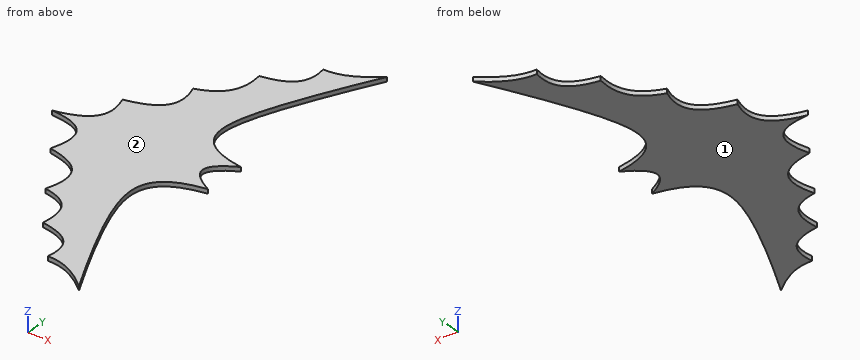
Autodesk Fusion 360 part; units mm, degrees
sketch "Sketch1" plane through (0, 0, 0) normal (0, 0, 1) x (1, 0, 0)
  spline S0 degree 5 poles (20, 5) (19.6208, 4.8) (18.8954, 4.4) (17.9067, 3.8) (16.7905, 3) (15.7547, 2) (15.1106, 1) (14.89, 0) (15.1106, -1) (15.7547, -2) (16.7905, -3) (17.9067, -3.8) (18.8954, -4.4) (19.6208, -4.8) (20, -5) knots 0 0 0 0 0 0 0.1 0.2 0.3 0.4 0.5 0.6 0.7 0.8 0.9 1 1 1 1 1 1
  spline S1 degree 5 poles (20, 5) (19.2712, 5.1081) (17.8733, 5.3538) (15.9554, 5.8111) (13.759, 6.5997) (11.6261, 7.8912) (10.1129, 9.4979) (9.2114, 11.428) (8.8832, 13.6833) (9.0671, 16.2602) (9.6928, 19.1509) (10.6903, 22.3442) (11.9999, 25.8244) (13.5744, 29.5733) (15.3779, 33.5733) (17.3852, 37.8091) (19.1413, 41.3771) (20.5394, 44.1509) (21.5072, 46.0431) (22, 47) knots 0 0 0 0 0 0 0.066667 0.133333 0.2 0.266667 0.333333 0.4 0.466667 0.533333 0.6 0.666667 0.733333 0.8 0.866667 0.933333 1 1 1 1 1 1
  spline S2 degree 5 poles (20, -5) (19.2712, -5.1081) (17.8733, -5.3538) (15.9554, -5.8111) (13.759, -6.5997) (11.6261, -7.8912) (10.1129, -9.4979) (9.2114, -11.428) (8.8832, -13.6833) (9.0671, -16.2602) (9.6928, -19.1509) (10.6903, -22.3442) (11.9999, -25.8244) (13.5744, -29.5733) (15.3779, -33.5733) (17.3852, -37.8091) (19.1413, -41.3771) (20.5394, -44.1509) (21.5072, -46.0431) (22, -47) knots 0 0 0 0 0 0 0.066667 0.133333 0.2 0.266667 0.333333 0.4 0.466667 0.533333 0.6 0.666667 0.733333 0.8 0.866667 0.933333 1 1 1 1 1 1
  spline S3 degree 5 poles (22, 47) (21.7727, 46.8021) (21.3189, 46.4146) (20.6399, 45.8581) (19.7383, 45.1666) (18.6179, 44.3921) (17.5049, 43.7166) (16.4, 43.1495) (15.3036, 42.6985) (14.2158, 42.3629) (13.136, 42.1358) (12.2781, 42.0345) (11.6378, 42.001) (11.2124, 41.9972) (11, 42) knots 0 0 0 0 0 0 0.1 0.2 0.3 0.4 0.5 0.6 0.7 0.8 0.9 1 1 1 1 1 1
  spline S4 degree 5 poles (22, -47) (21.7727, -46.8021) (21.3189, -46.4146) (20.6399, -45.8581) (19.7383, -45.1666) (18.6179, -44.3921) (17.5049, -43.7166) (16.4, -43.1495) (15.3036, -42.6985) (14.2158, -42.3629) (13.136, -42.1358) (12.2781, -42.0345) (11.6378, -42.001) (11.2124, -41.9972) (11, -42) knots 0 0 0 0 0 0 0.1 0.2 0.3 0.4 0.5 0.6 0.7 0.8 0.9 1 1 1 1 1 1
  spline S5 degree 5 poles (11, 42) (11.0567, 41.6874) (11.1508, 41.074) (11.2338, 40.1895) (11.2264, 39.0824) (11.0075, 37.8268) (10.5616, 36.7102) (9.8726, 35.7422) (8.9361, 34.9257) (7.7664, 34.252) (6.3831, 33.7089) (5.1205, 33.3698) (4.0916, 33.1657) (3.3698, 33.0516) (3, 33) knots 0 0 0 0 0 0 0.1 0.2 0.3 0.4 0.5 0.6 0.7 0.8 0.9 1 1 1 1 1 1
  spline S6 degree 5 poles (11, -42) (11.0567, -41.6874) (11.1508, -41.074) (11.2338, -40.1895) (11.2264, -39.0824) (11.0075, -37.8268) (10.5616, -36.7102) (9.8726, -35.7422) (8.9361, -34.9257) (7.7664, -34.252) (6.3831, -33.7089) (5.1205, -33.3698) (4.0916, -33.1657) (3.3698, -33.0516) (3, -33) knots 0 0 0 0 0 0 0.1 0.2 0.3 0.4 0.5 0.6 0.7 0.8 0.9 1 1 1 1 1 1
  spline S7 degree 5 poles (3, 33) (3.0488, 32.6643) (3.1298, 32.003) (3.2017, 31.0414) (3.1969, 29.8211) (3.0117, 28.4056) (2.6312, 27.1097) (2.0398, 25.9431) (1.2292, 24.9109) (0.2085, 24.0075) (-1.0064, 23.2232) (-2.1209, 22.683) (-3.0317, 22.3239) (-3.6718, 22.1046) (-4, 22) knots 0 0 0 0 0 0 0.1 0.2 0.3 0.4 0.5 0.6 0.7 0.8 0.9 1 1 1 1 1 1
  spline S8 degree 5 poles (3, -33) (3.0519, -32.6532) (3.1391, -31.9722) (3.2199, -30.9891) (3.2258, -29.756) (3.0522, -28.3533) (2.6811, -27.1017) (2.0958, -26.0139) (1.2865, -25.0975) (0.261, -24.3466) (-0.965, -23.749) (-2.0931, -23.3837) (-3.0168, -23.1691) (-3.6666, -23.052) (-4, -23) knots 0 0 0 0 0 0 0.1 0.2 0.3 0.4 0.5 0.6 0.7 0.8 0.9 1 1 1 1 1 1
  spline S9 degree 5 poles (-4, 22) (-3.8671, 21.6411) (-3.6275, 20.9356) (-3.3469, 19.9148) (-3.1327, 18.6296) (-3.149, 17.1578) (-3.4725, 15.8318) (-4.1248, 14.6617) (-5.1107, 13.6499) (-6.4105, 12.787) (-7.9976, 12.0604) (-9.4768, 11.5784) (-10.6963, 11.2692) (-11.5574, 11.0859) (-12, 11) knots 0 0 0 0 0 0 0.1 0.2 0.3 0.4 0.5 0.6 0.7 0.8 0.9 1 1 1 1 1 1
  spline S10 degree 5 poles (-4, -23) (-3.8615, -22.5957) (-3.6109, -21.8015) (-3.3142, -20.6538) (-3.0793, -19.2121) (-3.0716, -17.5674) (-3.3744, -16.0936) (-4.0114, -14.8039) (-4.9925, -13.7036) (-6.3007, -12.7834) (-7.91, -12.029) (-9.4177, -11.5468) (-10.6645, -11.249) (-11.5464, -11.0783) (-12, -11) knots 0 0 0 0 0 0 0.1 0.2 0.3 0.4 0.5 0.6 0.7 0.8 0.9 1 1 1 1 1 1
  spline S11 degree 5 poles (-12, 11) (-11.8671, 10.6411) (-11.6275, 9.9356) (-11.3469, 8.9148) (-11.1327, 7.6296) (-11.149, 6.1578) (-11.4725, 4.8318) (-12.1248, 3.6617) (-13.1107, 2.6499) (-14.4105, 1.787) (-15.9976, 1.0604) (-17.4768, 0.5784) (-18.6963, 0.2692) (-19.5574, 0.0859) (-20, 0) knots 0 0 0 0 0 0 0.1 0.2 0.3 0.4 0.5 0.6 0.7 0.8 0.9 1 1 1 1 1 1
  spline S12 degree 5 poles (-12, -11) (-11.8595, -10.5833) (-11.605, -9.7673) (-11.3024, -8.5952) (-11.0601, -7.1378) (-11.0439, -5.5036) (-11.3393, -4.0734) (-11.9708, -2.8631) (-12.9501, -1.8804) (-14.2612, -1.1149) (-15.8784, -0.5497) (-17.3964, -0.2443) (-18.653, -0.0926) (-19.5424, -0.0252) (-20, 0) knots 0 0 0 0 0 0 0.1 0.2 0.3 0.4 0.5 0.6 0.7 0.8 0.9 1 1 1 1 1 1
  point P0 (15, 0)
  point P1 (10, 10)
  point P2 (10, 20)
  point P3 (10, -10)
  point P4 (10, -20)
  point P5 (16, 43)
  point P6 (16, -43)
  point P7 (10, 36)
  point P8 (10, -36)
  point P9 (2, 26)
  point P10 (2, -26)
  point P11 (-4, 15)
  point P12 (-4, -15)
  point P13 (-12, 4)
  point P14 (-12, -3)
extrude "Extrude1" add sketch "Sketch1" along normal blind 1
CAD build for the part. Positions are in the model's coordinates, mm. Face numbers are marked on the shaded views. Give positions to 0.01 mm unless a question says otherwise; leave off trailing zeros.
(1) Saw through at A-A, the plane x = 17.5. State how many separate pieces and enclosed holes the cut face has, then the cut area to 3 significant figures.
(2) Drill centre lines: L1, parallel to X at y = 31, z = 0.6; L2, parallel to Y at x = -13, z = 0.4; L3, parallel to X at y = 28, z = 0.4. Where is each one in solid material? Low to high.
(3) Mould opens along Z. For the marked faces 1 and 2 say: released by +Z, released by -Z, zero draft, split by the parting line, or undercut.
Results found:
1. separate pieces: 4
1. enclosed holes: 0
1. area: 15.5 mm2
2. L1: x = 3.17 to 14.23
2. L2: y = -1.96 to 2.85
2. L3: x = 2.86 to 12.93
3. face 1: released by -Z
3. face 2: released by +Z
